Geometry check sheet. Reference: drawing and pictorial views, mm from the part's lowest x, y, z. A direction names the side the tool comes from. Give positions to 0.01 mm unless a question says otherwise; leave off trailing zeros. Order: outer loops, then holes, each group sorted by start corner. A loop starts at its lowest first (then second) coordinate and runs counter-clockwise, first axis right, second up.
Item 1: Sectioned sample at B-B on y = 12. Record the boundary of the cut face in (x, z).
Item 2: Gauge pin test, flat ends, axial feed: P1, Ø1.5, axis at y = 6, z = 7.5, coming from the +X side; P2, Ø5, axis at y = 10.5, z = 7.5, coming from the +X side; P3, Ø3.5, axis at x = 16.5, z = 12, coming from the +Y side. Record the tip position at first contact, or that the pin passes through.
Item 3: Release check for a two-part mould opening along Z. For the marked faces 3, 4, 5 and 6 record: released by +Z, released by -Z, zero draft, split by the parting line, or undercut.
Item 4: Sectioned sample at D-D on z = 6.25. Record the boundary of the cut face in (x, y), and give its area (3 significant figures).
Item 5: Material ranges on line 1 along Z through (x, y) = (14, 3.1); line 2 along Z through (x, y) = (1.5, 12); line 3 along Y through (x, z) = (9.75, 6.75), recorded low to high.
Item 6: Access from +Z, -Z, +X, -X, +Y, -Y to the whole of each face (thin tool, end or side, straight path). Record for the marked faces 1 and 2.
Item 7: Sectioned sample at A-A on z = 9. Record the boundary of the cut face in (x, y).
Item 8: Sectioned sample at C-C on x = 14. Record the boundary of the cut face in (y, z).
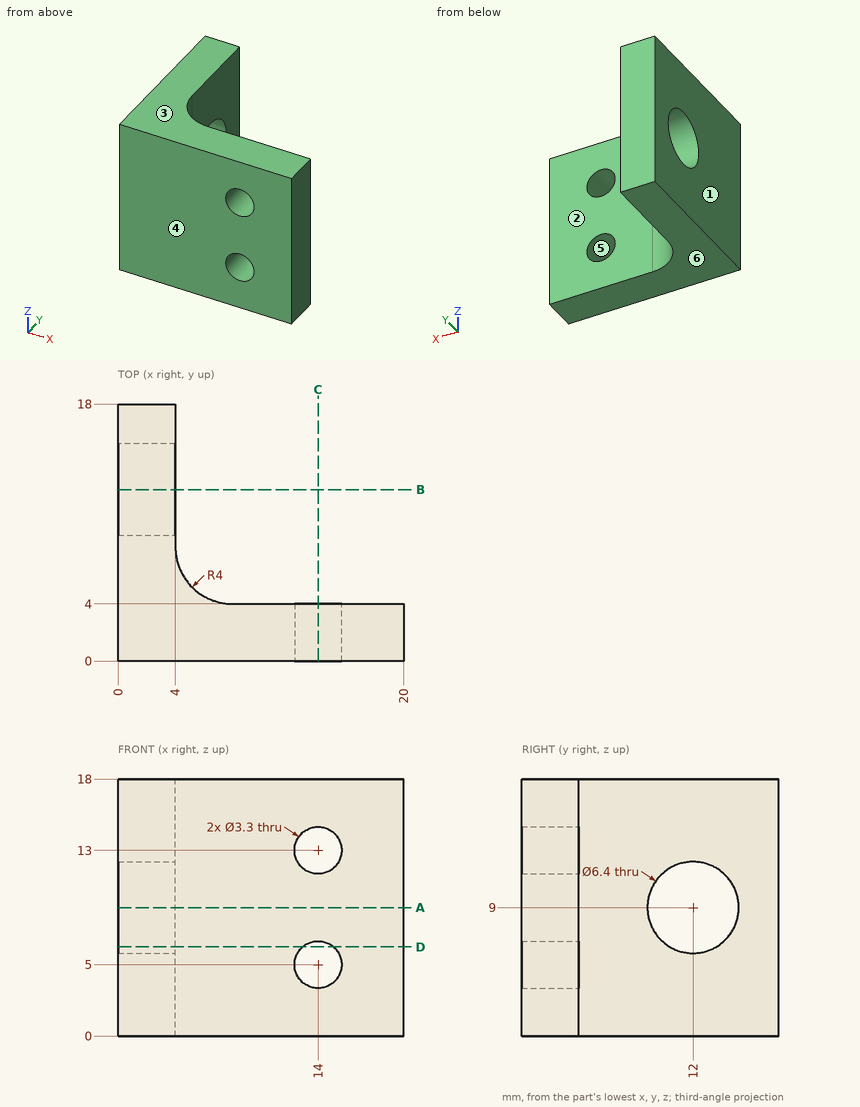
Report:
1. outline: (0, 0) - (4, 0) - (4, 5.8) - (0, 5.8) - close; (0, 12.2) - (4, 12.2) - (4, 18) - (0, 18) - close
2. P1: stops at x = 5.1
2. P2: stops at x = 4
2. P3: stops at y = 4
3. face 3: released by +Z
3. face 4: zero draft
3. face 5: undercut
3. face 6: released by -Z
4. outline: (0, 0) - (12.92, 0) - (12.92, 4) - (8, 4) arc R4 cw to (4, 8) - (4, 10.36) - (0, 10.36) - close; (0, 13.64) - (4, 13.64) - (4, 18) - (0, 18) - close; (15.08, 0) - (20, 0) - (20, 4) - (15.08, 4) - close
4. area: 118 mm2
5. line 1: z = 0 to 3.35, 6.65 to 11.35, 14.65 to 18
5. line 2: z = 0 to 5.8, 12.2 to 18
5. line 3: y = 0 to 4
6. face 1: +Z, -Z, -X, +Y, -Y
6. face 2: +Z, -Z, +X, +Y
7. outline: (0, 0) - (20, 0) - (20, 4) - (8, 4) arc R4 cw to (4, 8) - (4, 8.8) - (0, 8.8) - close; (0, 15.2) - (4, 15.2) - (4, 18) - (0, 18) - close
8. outline: (0, 0) - (4, 0) - (4, 3.35) - (0, 3.35) - close; (0, 6.65) - (4, 6.65) - (4, 11.35) - (0, 11.35) - close; (0, 14.65) - (4, 14.65) - (4, 18) - (0, 18) - close
